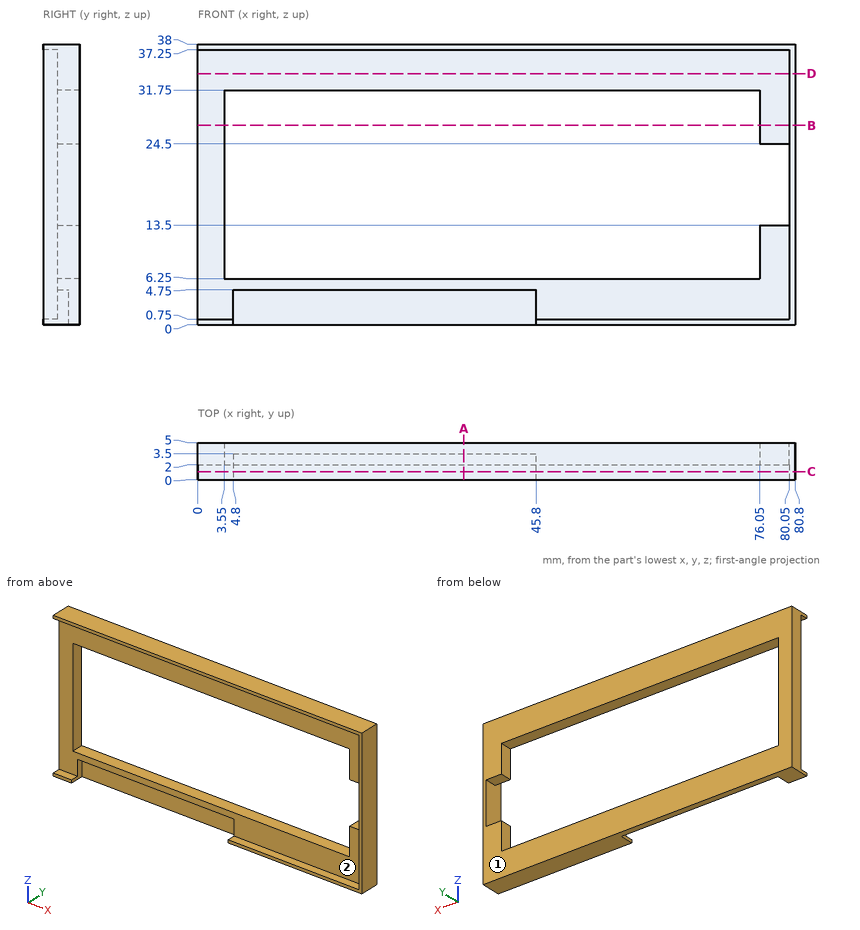
For this review, use the dimensioned drawing (mm, ordinates from the lowest corner) and the shaded views. Give positions to 0.01 mm unless a question says otherwise; leave off trailing zeros. Write each loop counter-clockwise with the first axis right and the second up, starting at its lowest first coordinate (ties: lowest second). Pieces come first, ordered by that corner, then holes. Notation, with made-up numbers: M 33.25,-5 L 42.25,-5 A31 cw 42.25,19 Z; hole C 21,76 d6. An arc over 180 degrees is marked long. Answer as a JSON object with one key per item and string values. Group by question number.
Item 1: Consider section A-A on x = 36. Write out the cut boundary in (y, z), plus the area to 3 significant figures.
Item 2: For pin 1 Ø11 at (x, z) = (44.5, 12.5) entering from -Y; pin 2 Ø1.6 at (x, y) = (30.5, 2.5) entering from -Z; pin 3 Ø5 at (x, z) = (22.5, 2) entering from -Y; pin 4 Ø1.6 at (x, y) = (44.5, 1) entering from -Z, all flat-tipped, find the tip position at first contact; note any pin that passes through.
Item 3: Consider section D-D on z = 34. Write out the cut boundary in (x, y), plus the area to 3 significant figures.
Item 4: Consider section B-B on z = 27. Write out the cut boundary in (x, y), plus the area to 3 significant figures.
Item 5: For probe 1 along X at (y, z) = (4.2, 11.5); probe 2 along Z at (x, y) = (46, 4.45); probe 3 along X at (y, z) = (3.8, 20.5), list the stretches that pass through material, from the lowest coordinate up. Write a range as [from, to].
Item 6: Draft analysis for pull direction Z (two halves, no side actions). For the marked faces 1 and 2, state which applies: +Z half, -Z half, draft (parallel to the pull), parting line (faces both ways), or undercut.
Item 7: Consider section C-C on y = 1.1. Write out the cut boundary in (x, z).
Check result:
{
 "1": {"outline": "M 0,37.25 L 2,37.25 L 2,31.75 L 5,31.75 L 5,38 L 0,38 Z; M 2,4.75 L 3.5,4.75 L 3.5,0 L 5,0 L 5,6.25 L 2,6.25 Z", "area": "31.9 mm^2"},
 "2": {"pin 1": "passes through", "pin 2": "stops at z = 4.75", "pin 3": "stops at y = 3.5", "pin 4": "stops at z = 37.25"},
 "3": {"outline": "M 0,2 L 80.05,2 L 80.05,0 L 80.8,0 L 80.8,5 L 0,5 Z", "area": "244 mm^2"},
 "4": {"outline": "M 0,2 L 3.55,2 L 3.55,5 L 0,5 Z; M 76.05,2 L 80.05,2 L 80.05,0 L 80.8,0 L 80.8,5 L 76.05,5 Z", "area": "26.4 mm^2"},
 "5": {"probe 1": "x = [0, 3.55], [76.05, 80.8]", "probe 2": "z = [0, 6.25], [31.75, 38]", "probe 3": "x = [0, 3.55], [80.05, 80.8]"},
 "6": {"face 1": "draft", "face 2": "undercut"},
 "7": {"outline": "M 0,0 L 4.8,0 L 4.8,0.75 L 0,0.75 Z; M 0,37.25 L 80.05,37.25 L 80.05,0.75 L 45.8,0.75 L 45.8,0 L 80.8,0 L 80.8,38 L 0,38 Z"}
}
